Part model, mm, in its own coordinate system. A direction names the side the tool comes from. Round coordinates to 2 decimals unless told otherwise and drop trailing zeros. Loops run counter-clockwise (first coordinate to the right, second up) from the corner with the lowest first, then second, coordinate; pieces in that order, holes last.
1) Band-saw the part on B-B, the plane x = -3. Write the cut outline in (y, z).
2) Band-saw the part on D-D, the plane z = 0.9. Write the cut outline in (x, y), then the cut area to 3 significant figures.
3) Band-saw the part on C-C, the plane y = 4.6. Write the cut outline in (x, z), then the cut area to 3 significant figures.
4) Mould opens along X. For faces 1 (the flat face through (0, 2, -2.5)), 2 (the flat face through (-5, 2, 0)), 3 (the flat face through (3, 2, -1)) say: +X half, -X half, draft (parallel to the pull), parting line (faces both ways), or undercut.
5) Drop flat-ended pins along their axis: P1, Ø1.8, axis at x = -2.24, z = 0, coming from the +Y side; P2, Ø1, axis at x = -3, z = -1, coming from the -Y side. Give the stop position or say it passes through.
6) Probe line 1 (X direction, y = 1.45, z = 0); line 2 (X direction, y = 0.5, z = 0.9); line 3 (Z direction, x = 2.25, y = 3.7). List the from-to ranges inside material, lowest first.
7) 3-axis set-ups, long thin cutter, end or side, ignore diameter. For faces 4 (the flat face through (0, 5, 0)), 5 (the flat face through (4, 2, 0)): which of +Z, -Z, +X, -X, +Y, -Y reach the whole face in a straight line?
8) Band-saw the part on A-A, the plane z = 0. Write the cut outline in (x, y), then the cut area to 3 significant figures.
from build123d import *

# Parameters (mm, degrees)
SKETCH1_W           = 10
SKETCH1_H           = 5
SKETCH1_R           = 1
SKETCH1_W_2         = 2
SKETCH1_H_2         = 2
BOSS_EXTRUDE2_DEPTH = 5


with BuildPart() as part:
    # Sketch1 → Boss-Extrude2 (new body)
    with BuildSketch(Plane(origin=(0, 0, 0), x_dir=(1, 0, 0), z_dir=(0, 1, 0))):
        Rectangle(SKETCH1_W, SKETCH1_H)
        with Locations(Location((-2.236067977, 0, 0), (0, 0, 270))):
            Circle(SKETCH1_R, mode=Mode.SUBTRACT)
        with Locations((3, 0)):
            Rectangle(SKETCH1_W_2, SKETCH1_H_2, mode=Mode.SUBTRACT)
    extrude(amount=BOSS_EXTRUDE2_DEPTH)


solid = part.part
Reported:
1. outline: (0, -2.5) - (5, -2.5) - (5, -0.65) - (0, -0.65) - close; (0, 0.65) - (5, 0.65) - (5, 2.5) - (0, 2.5) - close
2. outline: (-5, 0) - (-2.67, 0) - (-2.67, 5) - (-5, 5) - close; (-1.8, 0) - (2, 0) - (2, 5) - (-1.8, 5) - close; (4, 0) - (5, 0) - (5, 5) - (4, 5) - close
2. area: 35.6 mm2
3. outline: (-5, -2.5) - (5, -2.5) - (5, 2.5) - (-5, 2.5) - close; hole circle Ø2 at (-2.24, 0); hole (2, -1) - (4, -1) - (4, 1) - (2, 1) - close
3. area: 42.9 mm2
4. face 1: draft
4. face 2: -X half
4. face 3: undercut
5. P1: passes through
5. P2: stops at y = 0
6. line 1: x = -5 to -3.24, -1.24 to 2, 4 to 5
6. line 2: x = -5 to -2.67, -1.8 to 2, 4 to 5
6. line 3: z = -2.5 to -1, 1 to 2.5
7. face 4: +Z, -Z, +X, -X, +Y
7. face 5: +Y, -Y
8. outline: (-5, 0) - (-3.24, 0) - (-3.24, 5) - (-5, 5) - close; (-1.24, 0) - (2, 0) - (2, 5) - (-1.24, 5) - close; (4, 0) - (5, 0) - (5, 5) - (4, 5) - close
8. area: 30.0 mm2
